Autodesk Inventor part; units mm, degrees
ref_plane "YZ Plane" through (0, 0, 0) normal (1, 0, 0) x (0, 1, 0)
ref_plane "XZ Plane" through (0, 0, 0) normal (0, 1, 0) x (-1, 0, 0)
ref_plane "XY Plane" through (0, 0, 0) normal (0, 0, 1) x (1, 0, 0)
sketch "Sketch1" plane through (0, 0, 0) normal (0, 1, 0) x (-1, 0, 0)
  circle A0 centre (0, 0) radius 5
  circle A1 centre (0, 0) radius 7.5
  dimension "d0" = 10
  dimension "d1" = 15
extrude "Extrusion1" add sketch "Sketch1" against normal blind 2
extrude "Extrusion2" add sketch "Sketch1" against normal blind 112 contours A0
mirror "Mirror1" about plane through (0, -112, 0) normal (0, -1, 0) of "Extrusion2", "Extrusion1"
Part model, mm, in its own coordinate system. A direction names the side the tool comes from. Give positions to 0.01 mm unless a question says otherwise; leave off trailing zeros. Loops run counter-clockwise (first coordinate to the right, second up) from the corner with the lowest first, then second, coordinate; pieces in that order, holes last. Notation, with made-up numbers: M 9.25,-35 L 58.25,-35 A13 cw 58.25,-23 Z; hole C -27,-17.5 d3. An arc over 180 degrees is marked long. Return JSON: item names as keys, results as strings.
1) Pull direction Y, two halves, no side cores. Call faces 1 (the face through (1.08, -110.46, -4.88)), 2 (the face through (7.493, -223.014, -0.33)), 3 (the face through (0, 0, 0)): released by +Y, released by -Y, zero draft, split by the parting line, or undercut.
Calculated:
{"face 1": "undercut", "face 2": "zero draft", "face 3": "released by +Y"}
2) 3-axis set-ups, long thin cutter, end or side, ignore diameter. For faces 4 (the face through (0, -224, 0)), 5 (the face through (2, -222, -5)): which of +Z, -Z, +X, -X, +Y, -Y reach the whole face in a straight line?
Calculated:
{"face 4": "+Z, -Z, +X, -X, -Y", "face 5": "none"}
3) Saw through at B-B, the plane x = 0. List the corners of the cut face in (y, z).
Calculated:
{"outline": "M -224,-7.5 L -222,-7.5 L -222,-5 L -2,-5 L -2,-7.5 L 0,-7.5 L 0,7.5 L -2,7.5 L -2,5 L -222,5 L -222,7.5 L -224,7.5 Z"}
4) Saw through at C-C, the plane y = -168. List the corners of the cut face in (x, z), then the cut area to 3 significant figures.
Calculated:
{"outline": "C 0,0 d10", "area": "78.5 mm2"}
5) Saw through at A-A, the plane z = 0. List the corners of the cut face in (x, y).
Calculated:
{"outline": "M -7.5,-224 L 7.5,-224 L 7.5,-222 L 5,-222 L 5,-2 L 7.5,-2 L 7.5,0 L -7.5,0 L -7.5,-2 L -5,-2 L -5,-222 L -7.5,-222 Z"}
6) Drill centre lines: line 1 (Y direction, x = 5, z = 2); line 2 (X direction, y = -70.5, z = 0.5); line 3 (Z direction, x = 3.5, y = -28.5). Where is each one in solid material? Low to high.
Calculated:
{"line 1": "y = -224 to -222, -2 to 0", "line 2": "x = -4.97 to 4.97", "line 3": "z = -3.57 to 3.57"}
7) Flat gauge pins, fed straight in: pin 1 Ø8 at (x, y) = (0, -138) entering from -Z; pin 2 Ø3 at (y, z) = (-133.5, -4.5) entering from +X; pin 3 Ø8 at (y, z) = (-193.5, 1.5) entering from +X. Where does each tip first touch, or does it go through?
Calculated:
{"pin 1": "stops at z = -5", "pin 2": "stops at x = 4", "pin 3": "stops at x = 5"}
